from build123d import *

# Parameters (mm, degrees)
F1_DEPTH = 3.2385
F3_DEPTH = 5.9055
F4_R     = 1.7145
F5_DEPTH = 11.7475


with BuildPart() as f1:
    # F0 (on Top) → F1 (new body, symmetric)
    with BuildSketch(Plane.XY):
        with BuildLine():
            ThreePointArc((14.861846, 1.344079), (-14.907329, -0.672724), (14.9225, 0))
            ThreePointArc((14.9225, 0), (14.907329, 0.672724), (14.861846, 1.344079))
        make_face()
    extrude(amount=F1_DEPTH, both=True)

    # F2 (on Top) → F3 (join, symmetric)
    with BuildSketch(Plane.XY):
        with BuildLine():
            ThreePointArc((4.311158, 0.242977), (-4.316289, -0.121537), (4.318, 0))
            ThreePointArc((4.318, 0), (4.316289, 0.121537), (4.311158, 0.242977))
        make_face()
    extrude(amount=F3_DEPTH, both=True)

    # F4 (on Top) → F5 (join, symmetric)
    with BuildSketch(Plane.XY):
        Circle(F4_R)
    extrude(amount=F5_DEPTH, both=True)


solid = f1.part
Geometry: final body of the model. Coordinates: model frame, mm. A direction names the side the tool comes from. Give positions to 0.01 mm unless a question says otherwise; leave off trailing zeros. Write each loop counter-clockwise with the first axis right and the second up, starting at its lowest first coordinate (ties: lowest second). Pieces come first, ordered by that corner, then holes. Notation, with made-up numbers: (5, -33) -> (59, -33) arc R12 cw to (59, -25) -> close; hole circle Ø9 at (61.25, -27). An arc over 180 degrees is marked (long way). Answer in a Markdown table with one row per item.
(1) Section query D-D on x = 7.75. Return loops of the section in (y, z).
Answers below:
| item | result |
|---|---|
| outline | (-12.75, -3.24) -> (12.75, -3.24) -> (12.75, 3.24) -> (-12.75, 3.24) -> close |
(2) Section query A-A on x = 0. Return loops of the section in (y, z).
Answers below:
| item | result |
|---|---|
| outline | (-14.92, -3.24) -> (-4.32, -3.24) -> (-4.32, -5.91) -> (-1.71, -5.91) -> (-1.71, -11.75) -> (1.71, -11.75) -> (1.71, -5.91) -> (4.32, -5.91) -> (4.32, -3.24) -> (14.92, -3.24) -> (14.92, 3.24) -> (4.32, 3.24) -> (4.32, 5.91) -> (1.71, 5.91) -> (1.71, 11.75) -> (-1.71, 11.75) -> (-1.71, 5.91) -> (-4.32, 5.91) -> (-4.32, 3.24) -> (-14.92, 3.24) -> close |
(3) Pin query (flat end, axial travel): pin 1 (4 mm diameter, centred on x = -11, y = 5.5, fed in from +Z); pin 2 (1 mm diameter, centred on x = 0.5, z = -4.5, fed in from -Y); pin 3 (8 mm diameter, centred on y = -3, z = 6, fed in from +X); pin 4 (6 mm diameter, centred on x = -7.5, z = 8, fed in from -Y). Return the tip coordinate at first contact, or that it passes through.
Answers below:
| item | result |
|---|---|
| pin 1 | z = 3.24 |
| pin 2 | y = -4.32 |
| pin 3 | x = 14.92 |
| pin 4 | through |
(4) Ray query, line 1 along Z through (x, y) = (-12.5, -7); line 2 along Y through (x, z) = (5, -1.25); line 3 along X through (y, z) = (3.25, 0.25). Return the intervals inside material, ascending. Write a range as [from, to].
Answers below:
| item | result |
|---|---|
| line 1 | [-3.24, 3.24] |
| line 2 | [-14.06, 14.06] |
| line 3 | [-14.56, 14.56] |
(5) Section query B-B on y = -3. Return loops of the section in (x, z), then the cut area to 3 significant figures.
Answers below:
| item | result |
|---|---|
| outline | (-14.62, -3.24) -> (-3.11, -3.24) -> (-3.11, -5.91) -> (3.11, -5.91) -> (3.11, -3.24) -> (14.62, -3.24) -> (14.62, 3.24) -> (3.11, 3.24) -> (3.11, 5.91) -> (-3.11, 5.91) -> (-3.11, 3.24) -> (-14.62, 3.24) -> close |
| area | 222 mm^2 |
(6) Set-up query: faces 1 (the flat face through (0, 0, 11.748)), 2 (the cylindrical face through (-0.372, -1.674, -8.786)), 3 (the cylindrical face through (-4.317, 0.067, 4.591)). Return all of +Z, -Z, +X, -X, +Y, -Y with unobstructed straight access to the full face (end or side cutting, diameter ignored); none if empty.
Answers below:
| item | result |
|---|---|
| face 1 | +Z, +X, -X, +Y, -Y |
| face 2 | -Z |
| face 3 | +Z |
(7) Section query C-C on z = 4.75. Return loops of the section in (x, y).
Answers below:
| item | result |
|---|---|
| outline | (4.31, 0.24) arc R4.32 ccw (long way) to (4.32, 0) arc R4.32 ccw to start |
